Check sheet for the modelled part. Datum: model origin and axes. Units: mm. Give positions to 0.01 mm unless a question says otherwise; leave off trailing zeros. Order: outer loops, then holes, each group sorted by start corner. A loop starts at its lowest first (then second) coordinate and runs counter-clockwise, first axis right, second up. Notation, with made-up numbers: (54.5, 48) - (61.5, 48) arc R29 ccw to (61.5, 84) - close; hole circle Ø3 at (57.25, -17). An arc over 180 degrees is marked (long way). Answer in a Markdown table with one row per item.
Autodesk Inventor part; units mm, degrees
ref_plane "YZ Plane" through (0, 0, 0) normal (1, 0, 0) x (0, 1, 0)
ref_plane "XZ Plane" through (0, 0, 0) normal (0, 1, 0) x (-1, 0, 0)
ref_plane "XY Plane" through (0, 0, 0) normal (0, 0, 1) x (1, 0, 0)
sketch "Sketch1" plane through (0, 0, 0) normal (0, 1, 0) x (-1, 0, 0)
  circle A0 centre (0, 0) radius 13.5
  dimension "d0" = 27
extrude "Extrusion1" add sketch "Sketch1" along normal blind 5
sketch "Sketch2" plane through (0, 5, 0) normal (0, 1, 0) x (1, 0, 0)
  line L0 (7.5, -10) -> (7.5, 10)
  line L1 (7.5, 10) -> (-7.5, 10)
  circle A0 centre (0, 0) radius 13.5
  line L2 (-7.5, -10) -> (-6, -10)
  line L3 (-6, -10) -> (-6, -5)
  line L4 (-6, -5) -> (-7.5, -5)
  line L5 (-7.5, -5) -> (-7.5, -10)
  line L6 (-7.5, 5) -> (-6, 5)
  line L7 (-6, 5) -> (-6, 10)
  line L8 (-6, 10) -> (-7.5, 10)
  line L9 (-7.5, 10) -> (-7.5, 5)
  line L10 (-6, -3) -> (-4.5, -3)
  line L11 (-4.5, -3) -> (-4.5, 3)
  line L12 (-4.5, 3) -> (-6, 3)
  line L13 (-6, 3) -> (-6, -3)
  line L14 (-4.5, -10) -> (-3, -10)
  line L15 (-3, -10) -> (-3, -5)
  line L16 (-3, -5) -> (-4.5, -5)
  line L17 (-4.5, -5) -> (-4.5, -10)
  line L18 (-4.5, 5) -> (-3, 5)
  line L19 (-4.5, 10) -> (-4.5, 5)
  line L20 (-3, 5) -> (-3, 10)
  line L21 (-3, 10) -> (-4.5, 10)
  line L22 (-3, -3) -> (-1.5, -3)
  line L23 (-1.5, -3) -> (-1.5, 3)
  line L24 (-1.5, 3) -> (-3, 3)
  line L25 (-3, 3) -> (-3, -3)
  line L26 (-1.5, -10) -> (0, -10)
  line L27 (0, -10) -> (0, -5)
  line L28 (0, -5) -> (-1.5, -5)
  line L29 (-1.5, -5) -> (-1.5, -10)
  line L30 (-1.5, 5) -> (0, 5)
  line L31 (-1.5, 10) -> (-1.5, 5)
  line L32 (0, 5) -> (0, 10)
  line L33 (0, 10) -> (-1.5, 10)
  line L34 (0, -3) -> (1.5, -3)
  line L35 (1.5, -3) -> (1.5, 3)
  line L36 (1.5, 3) -> (0, 3)
  line L37 (0, 3) -> (0, -3)
  line L38 (1.5, -10) -> (3, -10)
  line L39 (3, -10) -> (3, -5)
  line L40 (3, -5) -> (1.5, -5)
  line L41 (1.5, -5) -> (1.5, -10)
  line L42 (1.5, 5) -> (3, 5)
  line L43 (1.5, 10) -> (1.5, 5)
  line L44 (3, 5) -> (3, 10)
  line L45 (3, 10) -> (1.5, 10)
  line L46 (3, -3) -> (4.5, -3)
  line L47 (4.5, -3) -> (4.5, 3)
  line L48 (4.5, 3) -> (3, 3)
  line L49 (3, 3) -> (3, -3)
  line L50 (4.5, -10) -> (6, -10)
  line L51 (6, -10) -> (6, -5)
  line L52 (6, -5) -> (4.5, -5)
  line L53 (4.5, -5) -> (4.5, -10)
  line L54 (4.5, 5) -> (6, 5)
  line L55 (4.5, 10) -> (4.5, 5)
  line L56 (6, 5) -> (6, 10)
  line L57 (6, 10) -> (4.5, 10)
  line L58 (6, -3) -> (7.5, -3)
  line L59 (7.5, -3) -> (7.5, 3)
  line L60 (7.5, 3) -> (6, 3)
  line L61 (6, 3) -> (6, -3)
  line L62 (-7.5, -10) -> (-7.5, 10)
  line L63 (7.5, -10) -> (-7.5, -10)
  point P0 (-4.5, 5)
  point P1 (-1.5, 5)
  point P2 (1.5, -5)
  point P3 (1.5, 5)
  point P4 (4.5, -5)
  point P5 (4.5, 5)
  point P6 (7.5, -5)
  point P7 (7.5, 5)
  dimension "d4" = 20
  dimension "d5" = 15
  dimension "d8" = 1.5
  dimension "d9" = 5
  dimension "d10" = 1.5
  dimension "d11" = 5
  dimension "d14" = 1.5
  dimension "d16" = 2
  dimension "d25" = 1.5
  dimension "d26" = 5
  dimension "d27" = 1.5
  dimension "d29" = 1.5
  dimension "d31" = 1.5
  dimension "d32" = 5
  dimension "d33" = 1.5
  dimension "d35" = 1.5
  dimension "d37" = 1.5
  dimension "d38" = 5
  dimension "d39" = 1.5
  dimension "d41" = 1.5
  dimension "d43" = 1.5
  dimension "d44" = 5
  dimension "d45" = 1.5
  dimension "d47" = 1.5
  dimension "d49" = 20
  dimension "d50" = 15
extrude "Extrusion2" cut sketch "Sketch2" against normal blind 5 contours L58 L61 L60 L0 | L50 L53 L52 L51 | L38 L41 L40 L39 | L56 L54 L55 L1 | L26 L29 L28 L27 | L44 L42 L43 L1 | L14 L17 L16 L15 | L32 L30 L31 L1 | L2 L5 L4 L3 | L20 L18 L19 L1 | L7 L6 L9 L1 | L13 L12 L11 L10 | L25 L24 L23 L22 | L37 L36 L35 L34 | L49 L48 L47 L46
sketch "Sketch3" plane through (0, 5, 0) normal (0, 1, 0) x (1, 0, 0)
  point P0 (0, 0)
sketch "Sketch4" plane through (0, 5, 0) normal (0, 1, 0) x (1, 0, 0)
  point P0 (0, 0)
sketch "Sketch5" plane through (0, 5, 0) normal (0, 1, 0) x (1, 0, 0)
  point P0 (0, 0)
sketch "Sketch6" plane through (0, 5, 0) normal (0, 1, 0) x (1, 0, 0)
  circle A0 centre (-11, 0) radius 1
  circle A1 centre (0, 0) radius 13.5
  circle A2 centre (11, 0) radius 1
  line L0 (0, -3) -> (0, 3)
  dimension "d53" = 2
  dimension "d54" = 11
  dimension "d55" = 2
  dimension "d56" = 11
extrude "Extrusion3" cut sketch "Sketch6" against normal blind 5 contours A0 | A2
properties part number "Acrylic_Seperator"
(1) Mould release check, pull along X, two halves, no side actions. Record for faces 1 (the cylindrical face through (2.93, 2.46, 13.18)), 2 (the flat face through (2, 3, 10)): pulls with the +X half, pulls with the -X half, needs draft (parallel to the pull), parting line crosses it, or undercut.
Geometry says:
| item | result |
|---|---|
| face 1 | parting line crosses it |
| face 2 | undercut |
(2) Cross-section at B-B, the plane x = 7. Record the cut outline in (y, z).
Geometry says:
| item | result |
|---|---|
| outline | (0, -11.54) - (5, -11.54) - (5, -3) - (0, -3) - close; (0, 3) - (5, 3) - (5, 11.54) - (0, 11.54) - close |
(3) Cross-section at D-D, the plane x = -11. Record the cut outline in (y, z).
Geometry says:
| item | result |
|---|---|
| outline | (0, -7.83) - (5, -7.83) - (5, -1) - (0, -1) - close; (0, 1) - (5, 1) - (5, 7.83) - (0, 7.83) - close |
(4) Gauge pin test, flat ends, axial feed: P1, Ø2.5, axis at y = 3, z = -7, coming from the -X side; P2, Ø1.6, axis at x = -4, y = 3.5, coming from the +Z side; P3, Ø1.2, axis at x = 2, y = 3, coming from the -Z side; P4, Ø1.6, axis at x = -1, y = 3, coming from the -Z side. Record the tip position at first contact, or that the pin passes through.
Geometry says:
| item | result |
|---|---|
| P1 | x = -12.21 |
| P2 | z = 13.12 |
| P3 | z = -13.43 |
| P4 | z = -13.5 |
(5) Cross-section at A-A, the plane z = 0. Give the number of separate pieces and of enclosed holes in the cut face, then the cut area to 3 significant figures.
Geometry says:
| item | result |
|---|---|
| separate pieces | 8 |
| enclosed holes | 0 |
| area | 77.5 mm² |
(6) Thickness scan on L1, parallel to X at y = 4.1, z = 9.25; L2, parallel to X at y = 4.45, z = 8.5; L3, parallel to Z at x = -5.75, y = 3.15. Record the ranges inside material, lowest first.
Geometry says:
| item | result |
|---|---|
| L1 | -9.83 to -7.5, -6 to -4.5, -3 to -1.5, 0 to 1.5, 3 to 4.5, 6 to 9.83 |
| L2 | -10.49 to -7.5, -6 to -4.5, -3 to -1.5, 0 to 1.5, 3 to 4.5, 6 to 10.49 |
| L3 | -12.21 to -3, 3 to 12.21 |
